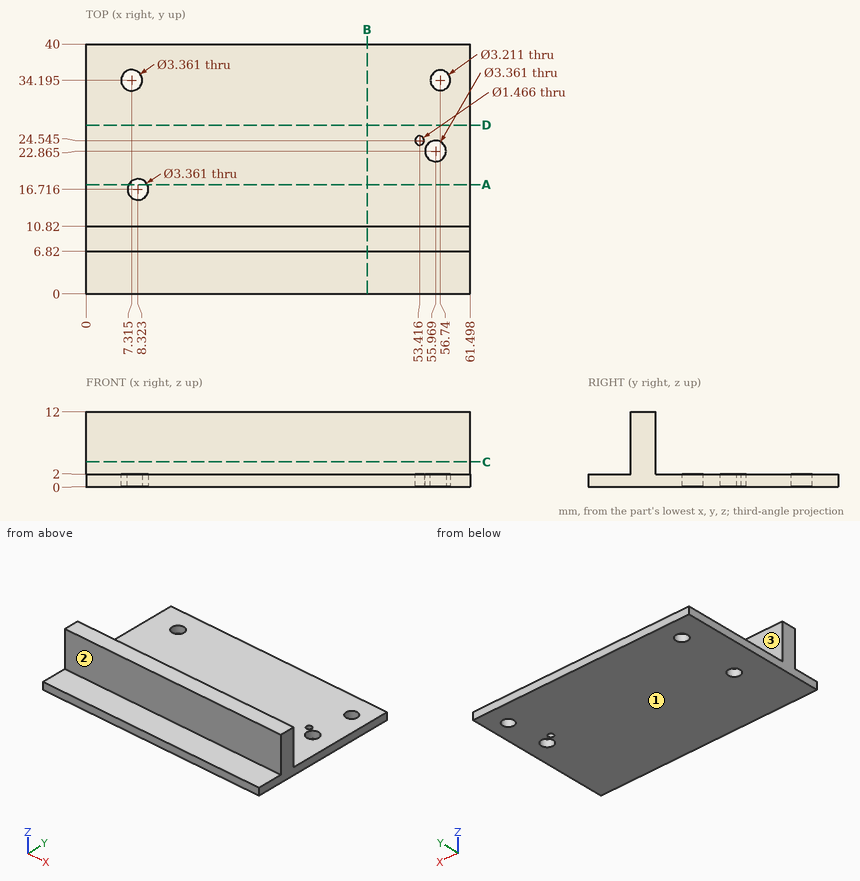
Input: dimensioned drawing with shaded views. Units: mm. Origin: part minimum x, y, z. A direction names the side the tool comes from. Give positions to 0.01 mm unless a question says otherwise; leave off trailing zeros. Loops run counter-clockwise (first coordinate to the right, second up) from the corner with the lowest first, then second, coordinate; pieces in that order, holes last. Notation, with made-up numbers: (56.25, -38.5) -> (60.25, -38.5) arc R19 ccw to (60.25, -3.5) -> close; hole circle Ø2 at (49, 4.5). An arc over 180 degrees is marked (long way). Return JSON: item names as keys, results as strings.
Item 1: Section B-B, the plane x = 45. Output: boundary loops of the cut face in (y, z).
Filled in:
{"outline": "(0, 0) -> (40, 0) -> (40, 2) -> (10.82, 2) -> (10.82, 12) -> (6.82, 12) -> (6.82, 2) -> (0, 2) -> close"}
Item 2: Access query for the marked faces 1, 2 and 3. Directions: +Z, -Z, +X, -X, +Y, -Y. A direction counts if a zero-diameter tool reaches every point of the face in a straight line with its end or side. Return the directions, or none.
Filled in:
{"face 1": "-Z, +X, -X, +Y, -Y", "face 2": "+Z, +X, -X, -Y", "face 3": "+Z, +X, -X, +Y"}
Item 3: Section A-A, the plane y = 17.5. Output: boundary loops of the cut face in (x, z), plus the area to 3 significant figures.
Filled in:
{"outline": "(0, 0) -> (6.84, 0) -> (6.84, 2) -> (0, 2) -> close; (9.81, 0) -> (61.5, 0) -> (61.5, 2) -> (9.81, 2) -> close", "area": "117 mm^2"}
Item 4: Section C-C, the plane z = 4. Output: boundary loops of the cut face in (x, y), plus the area to 3 significant figures.
Filled in:
{"outline": "(0, 6.82) -> (61.5, 6.82) -> (61.5, 10.82) -> (0, 10.82) -> close", "area": "246 mm^2"}
Item 5: Pin query (flat end, axial travel): P1, Ø5, axis at x = 26, z = 6.5, coming from the +Y side; P2, Ø10, axis at x = 40, y = 24.5, coming from the +Z side. Return the tip coordinate at first contact, or that it passes through.
Filled in:
{"P1": "y = 10.82", "P2": "z = 2"}
Item 6: Line query: line 1 (Y direction, x = 31, z = 6); line 2 (Z direction, x = 41, y = 24). Output: solid intervals per line, ascending.
Filled in:
{"line 1": "6.82 to 10.82", "line 2": "0 to 2"}
Item 7: Section D-D, the plane y = 27. Output: boundary loops of the cut face in (x, z).
Filled in:
{"outline": "(0, 0) -> (61.5, 0) -> (61.5, 2) -> (0, 2) -> close"}
